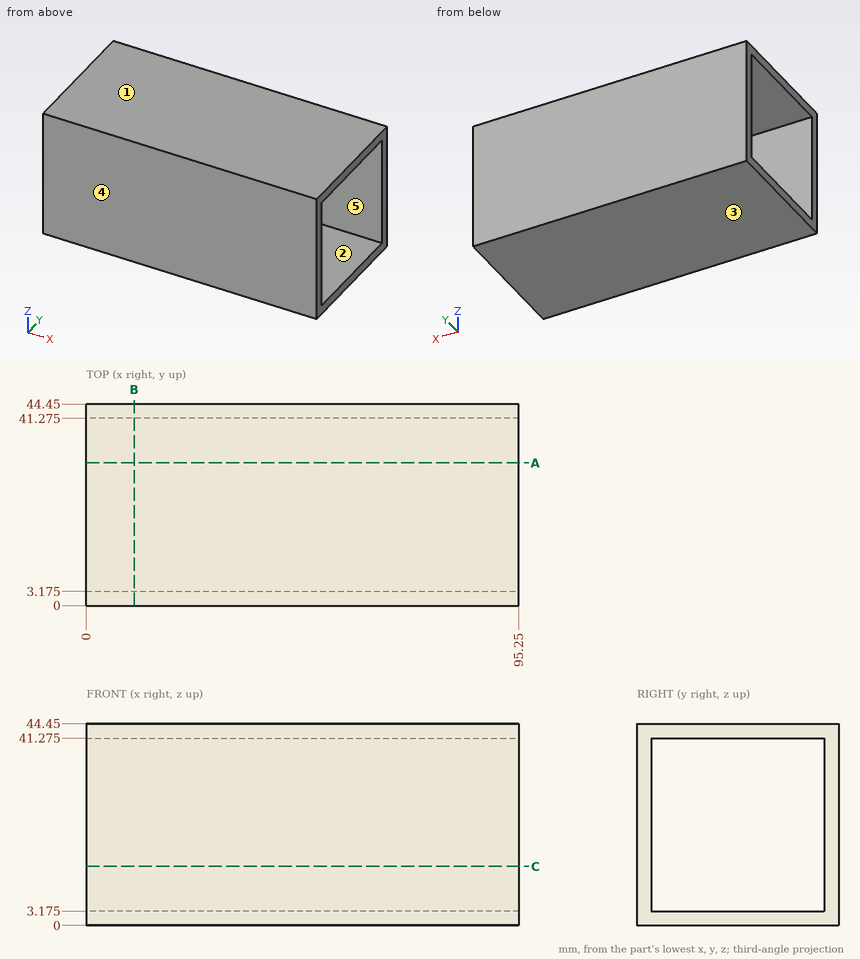
Design review of the part shown in the three views and the two pictorial views. Dimensions are in mm from the part's minimum x, y and z. A direction names the side the tool comes from. Give positions to 0.01 mm unless a question says otherwise; leave off trailing zeros. Loops run counter-clockwise (first coordinate to the right, second up) from the corner with the lowest first, then second, coordinate; pieces in that order, holes last. Notation, with made-up numbers: (-29.5, 21) -> (29.5, 21) arc R25 cw to (29.5, 48) -> close; hole circle Ø1 at (43.5, 53.25). An arc over 180 degrees is marked (long way). Put each result on its own line as item: value. Start each with the question number.
1. Wall thickness on probe 1 along Z at (x, y) = (51, 27) (3 decimals): over which ranges is the line inside the solid? List them lowest first.
2. For the marked faces 1 and 2, list the 3-axis set-ups (+Z, -Z, +X, -X, +Y, -Y) from which the entire face can be reached by the end or side of a thin tool; tool diameter is ignored.
3. We need section B-B on x = 10.5. State the section outline as (y, z) points (3 decimals), then the cut area to 3 significant figures.
4. Mouldability with a two-part tool opening along Y and no side actions: class the marked faces 3, 4 and 5 as released by +Y, released by -Y, zero draft, split by the parting line, or undercut.
5. We need section A-A on y = 31.5. State the section outline as (x, z) points (3 decimals).
Determined:
1. probe 1: 0 to 3.175, 41.275 to 44.45
2. face 1: +Z, +X, -X, +Y, -Y
2. face 2: +X, -X
3. outline: (0, 0) -> (44.45, 0) -> (44.45, 44.45) -> (0, 44.45) -> close; hole (3.175, 3.175) -> (41.275, 3.175) -> (41.275, 41.275) -> (3.175, 41.275) -> close
3. area: 524 mm^2
4. face 3: zero draft
4. face 4: released by -Y
4. face 5: undercut
5. outline: (0, 0) -> (95.25, 0) -> (95.25, 3.175) -> (0, 3.175) -> close; (0, 41.275) -> (95.25, 41.275) -> (95.25, 44.45) -> (0, 44.45) -> close
